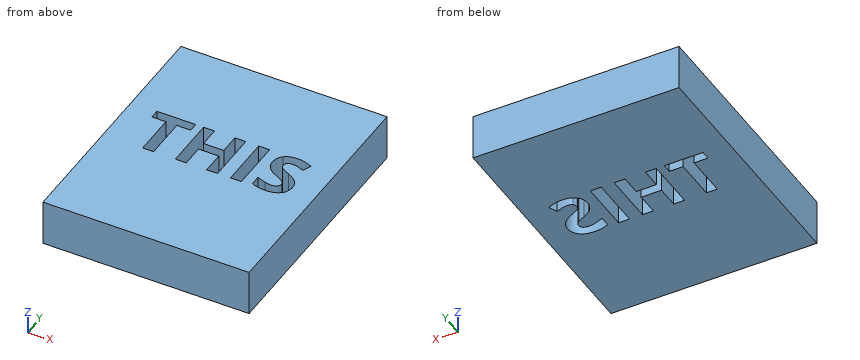
from build123d import *

# Parameters (mm, degrees)
F0_W     = 113.7968078256
F0_H     = 138.5442316532
F0_W_2   = 6.0173892501
F0_H_2   = 28.373014947
F1_DEPTH = 25.4


with BuildPart() as f1:
    # F0 (on Top) → F1 (new body)
    with BuildSketch(Plane.XY):
        Rectangle(F0_W, F0_H)
        Polygon((-28.96920121, 14.3365136363), (-28.96920121, -9.031325113), (-34.9865904601, -9.031325113), (-34.9865904601, 14.3365136363), (-42.6930714295, 14.3365136363), (-42.6930714295, 19.341689834), (-21.2689301366, 19.341689834), (-21.2689301366, 14.3365136363), align=None, mode=Mode.SUBTRACT)
        Polygon((6.3464774951, 19.341689834), (6.3464774951, -9.031325113), (0.3477179331, -9.031325113), (0.3477179331, 3.2145898521), (-10.8859839796, 3.2145898521), (-10.8859839796, -9.031325113), (-16.9033732297, -9.031325113), (-16.9033732297, 19.341689834), (-10.8859839796, 19.341689834), (-10.8859839796, 8.2197660498), (0.3477179331, 8.2197660498), (0.3477179331, 19.341689834), align=None, mode=Mode.SUBTRACT)
        with Locations((16.5151822392, 5.1551823605)):
            Rectangle(F0_W_2, F0_H_2, mode=Mode.SUBTRACT)
        with BuildLine():
            add(Edge.make_bspline(
                [(41.9384965735, 3.5343994975), (43.4133468799, 1.6248564692), (43.4133468799, -1.1509670549)],
                knots=[0, 0, 0, 1, 1, 1], degree=2))
            add(Edge.make_bspline(
                [(43.4133468799, -1.1509670549), (43.4133468799, -4.9948926955), (40.6468381999, -7.2087206291)],
                knots=[0, 0, 0, 1, 1, 1], degree=2))
            add(Edge.make_bspline(
                [(40.6468381999, -7.2087206291), (37.8803295199, -9.4225485627), (32.9558819705, -9.4225485627)],
                knots=[0, 0, 0, 1, 1, 1], degree=2))
            add(Edge.make_bspline(
                [(32.9558819705, -9.4225485627), (28.4102380788, -9.4225485627), (24.9202765117, -7.7086172593)],
                knots=[0, 0, 0, 1, 1, 1], degree=2))
            Line((24.9202765117, -7.7086172593), (24.9202765117, -2.1197108351))
            add(Edge.make_bspline(
                [(24.9202765117, -2.1197108351), (27.7892484761, -3.4051593126), (29.7795201528, -3.9267905789)],
                knots=[0, 0, 0, 1, 1, 1], degree=2))
            add(Edge.make_bspline(
                [(29.7795201528, -3.9267905789), (31.7697918294, -4.4484218452), (33.4216241726, -4.4484218452)],
                knots=[0, 0, 0, 1, 1, 1], degree=2))
            add(Edge.make_bspline(
                [(33.4216241726, -4.4484218452), (35.3963711091, -4.4484218452), (36.4551583817, -3.6939194779)],
                knots=[0, 0, 0, 1, 1, 1], degree=2))
            add(Edge.make_bspline(
                [(36.4551583817, -3.6939194779), (37.5139456543, -2.9394171106), (37.5139456543, -1.4428321681)],
                knots=[0, 0, 0, 1, 1, 1], degree=2))
            add(Edge.make_bspline(
                [(37.5139456543, -1.4428321681), (37.5139456543, -0.6107061005), (37.0482034523, 0.0413329823)],
                knots=[0, 0, 0, 1, 1, 1], degree=2))
            add(Edge.make_bspline(
                [(37.0482034523, 0.0413329823), (36.5824612503, 0.6933720651), (35.6789213783, 1.2926270317)],
                knots=[0, 0, 0, 1, 1, 1], degree=2))
            add(Edge.make_bspline(
                [(35.6789213783, 1.2926270317), (34.7753815064, 1.8918819983), (31.9995579824, 3.2145898521)],
                knots=[0, 0, 0, 1, 1, 1], degree=2))
            add(Edge.make_bspline(
                [(31.9995579824, 3.2145898521), (29.4038214431, 4.4379393694), (28.1028482255, 5.5619305503)],
                knots=[0, 0, 0, 1, 1, 1], degree=2))
            add(Edge.make_bspline(
                [(28.1028482255, 5.5619305503), (26.8018750079, 6.6859217311), (26.0256380045, 8.1825066736)],
                knots=[0, 0, 0, 1, 1, 1], degree=2))
            add(Edge.make_bspline(
                [(26.0256380045, 8.1825066736), (25.2494010011, 9.6790916161), (25.2494010011, 11.6724682408)],
                knots=[0, 0, 0, 1, 1, 1], degree=2))
            add(Edge.make_bspline(
                [(25.2494010011, 11.6724682408), (25.2494010011, 15.4418751291), (27.8016682682, 17.5936041024)],
                knots=[0, 0, 0, 1, 1, 1], degree=2))
            add(Edge.make_bspline(
                [(27.8016682682, 17.5936041024), (30.3539355353, 19.7453330758), (34.8561101548, 19.7453330758)],
                knots=[0, 0, 0, 1, 1, 1], degree=2))
            add(Edge.make_bspline(
                [(34.8561101548, 19.7453330758), (37.0668331404, 19.7453330758), (39.0757345051, 19.2237018095)],
                knots=[0, 0, 0, 1, 1, 1], degree=2))
            add(Edge.make_bspline(
                [(39.0757345051, 19.2237018095), (41.0846358698, 18.7020705432), (43.2767291673, 17.7519564511)],
                knots=[0, 0, 0, 1, 1, 1], degree=2))
            Line((43.2767291673, 17.7519564511), (41.3392416069, 13.0696948468))
            add(Edge.make_bspline(
                [(41.3392416069, 13.0696948468), (39.066419661, 14.0011792509), (37.5822545106, 14.3706680645)],
                knots=[0, 0, 0, 1, 1, 1], degree=2))
            add(Edge.make_bspline(
                [(37.5822545106, 14.3706680645), (36.0980893602, 14.7401568781), (34.6636033779, 14.7401568781)],
                knots=[0, 0, 0, 1, 1, 1], degree=2))
            add(Edge.make_bspline(
                [(34.6636033779, 14.7401568781), (32.9558819705, 14.7401568781), (32.0430272546, 13.9452901866)],
                knots=[0, 0, 0, 1, 1, 1], degree=2))
            add(Edge.make_bspline(
                [(32.0430272546, 13.9452901866), (31.1301725386, 13.1504234952), (31.1301725386, 11.8711849136)],
                knots=[0, 0, 0, 1, 1, 1], degree=2))
            add(Edge.make_bspline(
                [(31.1301725386, 11.8711849136), (31.1301725386, 11.0763182222), (31.4996613522, 10.4832731516)],
                knots=[0, 0, 0, 1, 1, 1], degree=2))
            add(Edge.make_bspline(
                [(31.4996613522, 10.4832731516), (31.8691501658, 9.890228081), (32.6733317013, 9.3375473346)],
                knots=[0, 0, 0, 1, 1, 1], degree=2))
            add(Edge.make_bspline(
                [(32.6733317013, 9.3375473346), (33.4775132368, 8.7848665882), (36.4831029138, 7.350380606)],
                knots=[0, 0, 0, 1, 1, 1], degree=2))
            add(Edge.make_bspline(
                [(36.4831029138, 7.350380606), (40.4636462671, 5.4439425257), (41.9384965735, 3.5343994975)],
                knots=[0, 0, 0, 1, 1, 1], degree=2))
        make_face(mode=Mode.SUBTRACT)
    extrude(amount=F1_DEPTH)


solid = f1.part
The model under review builds one solid part; all positions refer to its coordinate system, in mm. Coordinates: 2 decimals unless noted, no trailing zeros. Answer in a Markdown table with one row per item.
(1) Consider section A-A (z = 13). State how many separate pieces and enclosed holes the cut face has, plus the area to 3 significant figures.
Answers:
| item | result |
|---|---|
| separate pieces | 1 |
| enclosed holes | 4 |
| area | 14,600 mm² |
(2) Insertion check: pin 1 (4 mm diameter, centred on x = -8.5, y = 5.5, fed in from -Z). The pin has a flat end and moves straight along its axis. Give the tip position at first contact, or say it passes through.
Answers:
| item | result |
|---|---|
| pin 1 | through |
(3) Wall thickness on line 1 along X through (y, z) = (-7, 3.75); line 2 along Y through (x, z) = (30.5, 21); line 3 along Y through (x, z) = (35, 20.5): over which ranges is each line inside the solid? List them lowest first.
Answers:
| item | result |
|---|---|
| line 1 | -56.9 to -34.99, -28.97 to -16.9, -10.89 to 0.35, 6.35 to 13.51, 19.52 to 24.92, 40.9 to 56.9 |
| line 2 | -69.27 to -9.29, -4.1 to 3.97, 19.1 to 69.27 |
| line 3 | -69.27 to -9.32, -4.3 to 1.7, 8.07 to 14.74, 19.74 to 69.27 |
